CAD build for the part. Positions are in the model's coordinates, mm. Face numbers are marked on the shaded views. Give positions to 0.01 mm unless a question says otherwise; leave off trailing zeros. Write each loop counter-clockwise with the first axis right and the second up, starting at its lowest first coordinate (ties: lowest second). Pieces come first, ordered by that corner, then holes. Notation, with made-up numbers: (-22, 53.5) - (18, 53.5) arc R12 ccw to (18, 64.5) - close; hole circle Ø4 at (71.25, 45.25). An arc over 180 degrees is marked (long way). Answer as a JSON object with one key per item and string values.
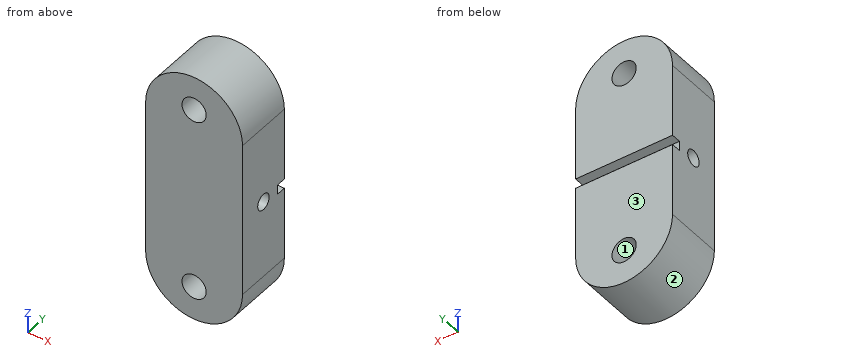
from build123d import *

# Parameters (mm, degrees)
SKETCH1_W               = 20
SKETCH1_H               = 12
BOSS_EXTRUDE1_DEPTH     = 26.035
M6X1_0_TAPPED_HOLE1_D   = 5
DELETEFACE1_START       = -6
DELETEFACE1_OUTLINE_R   = 2.5
DELETEFACE1_DEPTH       = 12
CUT_EXTRUDE1_DEPTH      = 29.527552033
CUT_EXTRUDE1_DEPTH_BACK = 29.527552033
SKETCH4_W               = 2
SKETCH4_H               = 2
M4X0_7_TAPPED_HOLE1_D   = 3.3
FILLET1_RADIUS          = 10
FILLET1_LENGTH          = 12
FILLET2_RADIUS          = 10
FILLET2_LENGTH          = 12


# Read off the part's stored shape, not the designer's step: DeleteFace1
with BuildPart() as part:
    # Sketch1 → Boss-Extrude1 (new, symmetric)
    with BuildSketch(Plane.XY):
        Rectangle(SKETCH1_W, SKETCH1_H)
    extrude(amount=BOSS_EXTRUDE1_DEPTH, both=True)

    # M6x1.0 Tapped Hole1 (through all)
    with Locations(Plane(origin=(0, 6, 0), x_dir=(1, 0, 0), z_dir=(0, 1, 0))):
        with Locations((0, -19.035), (0, 0), (0, 19.035)):
            Hole(M6X1_0_TAPPED_HOLE1_D / 2)

    # DeleteFace1 outline → DeleteFace1 (add)
    with BuildSketch(Plane(origin=(0, 0, 0), x_dir=(1, 0, 0), z_dir=(0, 1, 0)).offset(DELETEFACE1_START)):
        Circle(DELETEFACE1_OUTLINE_R)
    extrude(amount=DELETEFACE1_DEPTH)

    # Sketch4 → Cut-Extrude1 (cut, two sides: drawn at the far end of the back side and taken through both)
    with BuildSketch(Plane(origin=(0, 0, 0), x_dir=(0, 0, -1), z_dir=(1, 0, 0)).offset(-CUT_EXTRUDE1_DEPTH_BACK)):
        with Locations((0, 5)):
            Rectangle(SKETCH4_W, SKETCH4_H)
    extrude(amount=CUT_EXTRUDE1_DEPTH + CUT_EXTRUDE1_DEPTH_BACK, mode=Mode.SUBTRACT)

    # M4x0.7 Tapped Hole1 (through all)
    with Locations(Plane.ZY.offset(10)):
        with Locations((0, 0)):
            Hole(M4X0_7_TAPPED_HOLE1_D / 2)

    # Fillet1: full round fillet: the end face becomes a half cylinder, R = half its width
    fillet1_face = Plane((0, 0, -26.035), x_dir=(0, -1, 0), z_dir=(0, 0, -1))  # on the end face: x along it, z out of the body
    fillet1_slab = fillet1_face.offset(-FILLET1_RADIUS / 2) * Box(FILLET1_LENGTH, 2 * FILLET1_RADIUS, FILLET1_RADIUS, mode=Mode.PRIVATE)  # the body's end, R deep
    fillet1_round = Plane((0, 0, -16.035), x_dir=(0, 0, -1), z_dir=(0, -1, 0)) * Cylinder(FILLET1_RADIUS, FILLET1_LENGTH, mode=Mode.PRIVATE)  # its axis R under the face
    add(fillet1_slab - fillet1_round, mode=Mode.SUBTRACT)

    # Fillet2: full round fillet: the end face becomes a half cylinder, R = half its width
    fillet2_face = Plane((0, 0, 26.035), x_dir=(0, 1, 0), z_dir=(0, 0, 1))  # on the end face: x along it, z out of the body
    fillet2_slab = fillet2_face.offset(-FILLET2_RADIUS / 2) * Box(FILLET2_LENGTH, 2 * FILLET2_RADIUS, FILLET2_RADIUS, mode=Mode.PRIVATE)  # the body's end, R deep
    fillet2_round = Plane((0, 0, 16.035), x_dir=(0, 0, 1), z_dir=(0, 1, 0)) * Cylinder(FILLET2_RADIUS, FILLET2_LENGTH, mode=Mode.PRIVATE)  # its axis R under the face
    add(fillet2_slab - fillet2_round, mode=Mode.SUBTRACT)


solid = part.part
(1) Flat gauge pins, fed straight in: P1, Ø3, axis at x = 0, z = 19.035, coming from the +Y side; P2, Ø2, axis at x = 3.5, y = 5.5, coming from the -Z side; P3, Ø1.5, axis at x = -5.5, y = -3, coming from the +Z side; P4, Ø1, axis at x = 2, y = 5, coming from the +Z side. Where does each tip first touch, or does it go through?
Answer key:
{"P1": "passes through", "P2": "stops at z = -25.72", "P3": "stops at z = 24.83", "P4": "stops at z = 25.92"}
(2) Pull direction X, two halves, no side cores. Call the marked faces 1, 2 and 3: pulls with the +X half, pulls with the -X half, needs draft (parallel to the pull), parting line crosses it, or undercut.
Answer key:
{"face 1": "undercut", "face 2": "parting line crosses it", "face 3": "needs draft"}
(3) Saw through at D-D, the plane x = -6.25. Give the cut face in (y, z).
Answer key:
{"outline": "(-6, -23.84) - (6, -23.84) - (6, -1) - (4, -1) - (4, 1) - (6, 1) - (6, 23.84) - (-6, 23.84) - close; hole circle Ø3.3 at (0, 0)"}
(4) Probe L1, parallel to Z at x = 0, y = -2.5 (3 decimals); L2, parallel to Y at x = 3.75, z = 0; L3, parallel to Z at x = 0, y = 1 (3 decimals). List the from-to ranges inside material, lowest first. Write a range as [from, to].
Answer key:
{"L1": "z = [-26.035, -21.535], [-16.535, 16.535], [21.535, 26.035]", "L2": "y = [-6, -1.65], [1.65, 4]", "L3": "z = [-26.035, -21.535], [-16.535, -1.312], [1.312, 16.535], [21.535, 26.035]"}
(5) Saw through at B-B, the plane z = 0. Give the cut face in (x, y), and give its area (3 significant figures).
Answer key:
{"outline": "(-10, -6) - (10, -6) - (10, -1.65) - (-10, -1.65) - close; (-10, 1.65) - (10, 1.65) - (10, 4) - (-10, 4) - close", "area": "134 mm²"}
(6) Saw through at A-A, the plane x = 0. Give the cut face in (y, z) (3 decimals), and give its area (3 significant figures).
Answer key:
{"outline": "(-6, -26.035) - (6, -26.035) - (6, -21.535) - (-6, -21.535) - close; (-6, -16.535) - (6, -16.535) - (6, -1) - (4, -1) - (4, 1) - (6, 1) - (6, 16.535) - (-6, 16.535) - close; (-6, 21.535) - (6, 21.535) - (6, 26.035) - (-6, 26.035) - close; hole circle Ø3.3 at (0, 0)", "area": "492 mm²"}
(7) Saw through at C-C, the plane y = 0. Give the cut face in (x, z) (3 decimals), and give its area (3 significant figures).
Answer key:
{"outline": "(-10, -16.035) arc R10 ccw to (10, -16.035) - (10, -1.65) - (-10, -1.65) - close; (-10, 1.65) - (10, 1.65) - (10, 16.035) arc R10 ccw to (-10, 16.035) - close; hole circle Ø5 at (0, -19.035); hole circle Ø5 at (0, 19.035)", "area": "850 mm²"}
